For this review, take the finished solid that the model builds, in its own axes (mm). Round coordinates to 2 decimals unless told otherwise and drop trailing zeros. Order: outer loops, then holes, each group sorted by start corner. A loop starts at its lowest first (then second) coordinate and runs counter-clockwise, first axis right, second up. Notation, with made-up numbers: (-30, 45.25) - (10, 45.25) arc R17 cw to (10, 73.25) - close; hole circle Ø1 at (36.5, -25). An arc over 180 degrees is marked (long way). Write each question's results on one line, items separated by ' | '. Start each with the question number.
(1) Take a section at C-C, the plane z = 2.5. Give the number of separate pieces and of enclosed holes in the cut face, plus the area to 3 significant figures.
(2) Insertion check: pin 1 Ø8 at (x, y) = (-16.5, 3.5) entering from -Z; pin 2 Ø0.9 at (y, z) = (13, 2) entering from -X; pin 3 Ø0.9 at (x, z) = (13, 1.5) entering from -Y; pin 4 Ø0.9 at (x, z) = (17.5, 2) entering from +Y. Each pin has a flat end and moves straight along its axis. Give the tip position at first contact, or say it passes through.
(3) Draft analysis for pull direction Y (two halves, no side actions). For faces 1 (the cylindrical face through (-2.728, 20.777, 1.565)), 2 (the flat face through (12, 13.891, 2)), 3 (the flat face through (0, 5, 0)), state which applies: pulls with the +Y half, pulls with the -Y half, needs draft (parallel to the pull), parting line crosses it, or undercut.
(4) Take a section at A-A, the plane x = 0. Give the boundary of the cut face in (y, z) (3 decimals).
(5) Take a section at D-D, the plane x = 17. Give the boundary of the cut face in (y, z) (3 decimals), plus the area to 3 significant figures.
(6) For L1, parallel to Y at x = 0, z = 1.1 (3 decimals); L2, parallel to Y at x = -1, z = 1.4; L3, parallel to X at y = -2, z = 2.85, list the stretches that pass through material, from the lowest coordinate up. Write a range as from..to.
```python
from build123d import *

# Parameters (mm, degrees)
SKETCH1_R              = 20.955
SKETCH1_W              = 2.9972
SKETCH1_H              = 2.9972
BOSS_EXTRUDE1_DEPTH    = 3.175
CUT_EXTRUDE1_OUTLINE_R = 4.28625
CUT_EXTRUDE1_DEPTH     = 3.175


# Read off the part's stored shape, not the designer's step: Cut-Extrude1
with BuildPart() as part:
    # Sketch1 → Boss-Extrude1 (new body)
    with BuildSketch(Plane.XY):
        Circle(SKETCH1_R)
        with Locations((0, 17.526)):
            Rectangle(SKETCH1_W, SKETCH1_H, mode=Mode.SUBTRACT)
        with Locations((0, -17.526)):
            Rectangle(SKETCH1_W, SKETCH1_H, mode=Mode.SUBTRACT)
        with Locations((-17.526, 0)):
            Rectangle(SKETCH1_W, SKETCH1_H, mode=Mode.SUBTRACT)
        with Locations((17.526, 0)):
            Rectangle(SKETCH1_W, SKETCH1_H, mode=Mode.SUBTRACT)
        with Locations((-12.392753447, 12.392753447)):
            Rectangle(SKETCH1_W, SKETCH1_H, mode=Mode.SUBTRACT)
        with Locations((12.392753447, 12.392753447)):
            Rectangle(SKETCH1_W, SKETCH1_H, mode=Mode.SUBTRACT)
        with Locations((-12.392753447, -12.392753447)):
            Rectangle(SKETCH1_W, SKETCH1_H, mode=Mode.SUBTRACT)
        with Locations((12.392753447, -12.392753447)):
            Rectangle(SKETCH1_W, SKETCH1_H, mode=Mode.SUBTRACT)
    extrude(amount=BOSS_EXTRUDE1_DEPTH)

    # Cut-Extrude1 outline → Cut-Extrude1 (cut)
    with BuildSketch(Plane.XY):
        Circle(CUT_EXTRUDE1_OUTLINE_R)
    extrude(amount=CUT_EXTRUDE1_DEPTH, mode=Mode.SUBTRACT)


solid = part.part
```
Results below:
1) separate pieces: 1 | enclosed holes: 9 | area: 1,250 mm^2
2) pin 1: stops at z = 0 | pin 2: stops at x = -16.78 | pin 3: stops at y = -16.78 | pin 4: stops at y = 12.18
3) face 1: parting line crosses it | face 2: undercut | face 3: needs draft
4) outline: (-20.955, 0) - (-19.025, 0) - (-19.025, 3.175) - (-20.955, 3.175) - close; (-16.027, 0) - (-4.286, 0) - (-4.286, 3.175) - (-16.027, 3.175) - close; (4.286, 0) - (16.027, 0) - (16.027, 3.175) - (4.286, 3.175) - close; (19.025, 0) - (20.955, 0) - (20.955, 3.175) - (19.025, 3.175) - close
5) outline: (-12.252, 0) - (-1.499, 0) - (-1.499, 3.175) - (-12.252, 3.175) - close; (1.499, 0) - (12.252, 0) - (12.252, 3.175) - (1.499, 3.175) - close | area: 68.3 mm^2
6) L1: y = -20.955..-19.025, -16.027..-4.286, 4.286..16.027, 19.025..20.955 | L2: y = -20.93..-19.02, -16.03..-4.17, 4.17..16.03, 19.02..20.93 | L3: x = -20.86..-3.79, 3.79..20.86
